Autodesk Inventor part; units mm, degrees
ref_plane "YZ Plane" through (0, 0, 0) normal (1, 0, 0) x (0, 1, 0)
ref_plane "XZ Plane" through (0, 0, 0) normal (0, 1, 0) x (-1, 0, 0)
ref_plane "XY Plane" through (0, 0, 0) normal (0, 0, 1) x (1, 0, 0)
sketch "Sketch1" plane through (0, 0, 0) normal (0, 0, 1) x (1, 0, 0)
  circle A0 centre (0, 0) radius 4.826
  dimension "d7" = 9.652
extrude "Extrusion1" add sketch "Sketch1" along normal blind 27.94
sketch "Sketch2" plane through (0, 0, 27.94) normal (0, 0, 1) x (1, 0, 0)
  arc A0 (2.0632, 4.3627) -> (-1.7468, 4.4988) centre (0, 0) ccw
  circle A1 centre (0, 0) radius 4.826
  line L0 (-1.7468, 4.4988) -> (-1.7468, 2.5938)
  line L1 (-1.7468, 2.5938) -> (2.0632, 2.5938)
  line L2 (2.0632, 2.5938) -> (2.0632, 4.3627)
  dimension "d8" = 3.81
  dimension "d9" = 1.905
extrude "Extrusion2" add sketch "Sketch2" along normal blind 19.05 contours L2 L1 L0 A0
sketch "Sketch3" plane through (0, 0, 0) normal (0, 0, -1) x (-1, 0, 0)
  circle A0 centre (0, 0) radius 1.905
  dimension "d6" = 3.81
extrude "Extrusion3" add sketch "Sketch3" along normal blind 4.572
properties part number "emcoder_coupler"
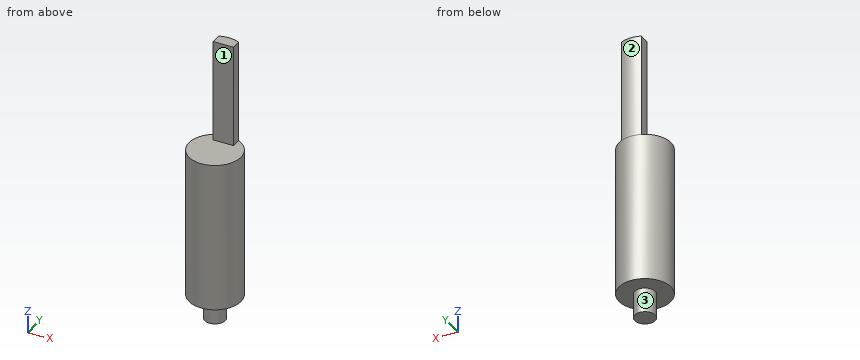
Verification items for the finished model (mm, model axes). Face numbers are marked on the shaded views. A direction names the side the tool comes from. Coordinates: 2 decimals unless noted, no trailing zeros. Order: outer loops, then holes, each group sorted by start corner. A loop starts at its lowest first (then second) coordinate and runs counter-clockwise, first axis right, second up. Notation, with made-up numbers: (58, -12) - (95, -12) arc R18 ccw to (95, -1) - close; hole circle Ø8 at (77.25, 0). An arc over 180 degrees is marked (long way). Return JSON: item names as keys, results as strings.
(1) Access from +Z, -Z, +X, -X, +Y, -Y to the whole of each face (thin tool, end or side, straight path). Record for the marked faces 1, 2 and 3.
Filled sheet:
{"face 1": "+Z, +X, -X, -Y", "face 2": "+Z, -Z, +Y", "face 3": "-Z"}
(2) Section check C-C, the plane z = 27. Record the cut outline in (x, y).
Filled sheet:
{"outline": "circle Ø9.65 at (0, 0)"}
(3) Go/stop test with flat-tipped pins: pin 1 (1 mm diameter, centred on y = 4, z = 36.5, fed in from -X); pin 2 (4 mm diameter, centred on x = -3, y = -3, fed in from -Z); pin 3 (1 mm diameter, centred on x = 2.5, y = -4, fed in from +Z); pin 4 (4 mm diameter, centred on x = -4, z = 32, fed in from -Y). Record where each tip stops, or that it passes through.
Filled sheet:
{"pin 1": "stops at x = -1.75", "pin 2": "stops at z = 0", "pin 3": "stops at z = 27.94", "pin 4": "passes through"}
(4) Section check D-D, the plane x = -3.25. Record the cut outline in (y, z).
Filled sheet:
{"outline": "(-3.57, 0) - (3.57, 0) - (3.57, 27.94) - (-3.57, 27.94) - close"}
(5) Thickness scan on line 1 along Z through (x, y) = (-4, -2); line 2 along X through (y, z) = (4.25, 39.5); line 3 along Z through (x, y) = (-0.25, -0.75). Record the ranges inside material, lowest first.
Filled sheet:
{"line 1": "z = 0 to 27.94", "line 2": "x = -1.75 to 2.06", "line 3": "z = -4.57 to 27.94"}
(6) Section check A-A, the plane x = 0. Record the cut outline in (y, z) (3 decimals).
Filled sheet:
{"outline": "(-4.826, 0) - (-1.905, 0) - (-1.905, -4.572) - (1.905, -4.572) - (1.905, 0) - (4.826, 0) - (4.826, 46.99) - (2.594, 46.99) - (2.594, 27.94) - (-4.826, 27.94) - close"}
(7) Section check B-B, the plane y = 0. Record the cut outline in (x, z) (3 decimals).
Filled sheet:
{"outline": "(-4.826, 0) - (-1.905, 0) - (-1.905, -4.572) - (1.905, -4.572) - (1.905, 0) - (4.826, 0) - (4.826, 27.94) - (-4.826, 27.94) - close"}
